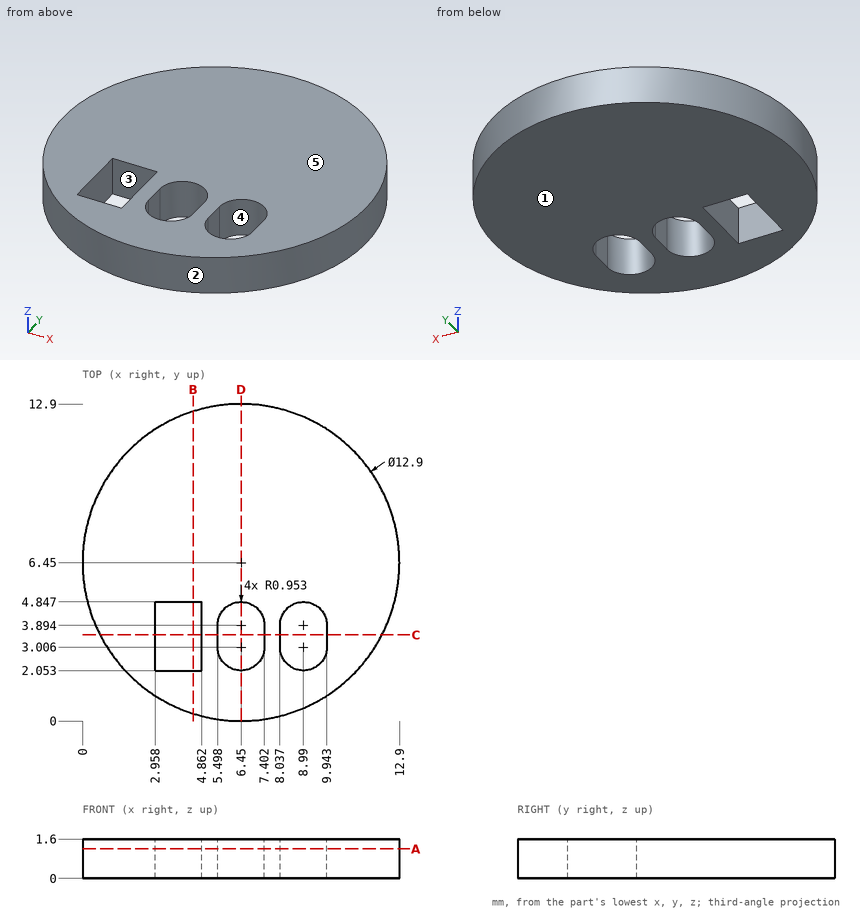
Print and shaded views of the part. All mm, measured from the part's lowest x, y and z. A direction names the side the tool comes from. Coordinates: 2 decimals unless noted, no trailing zeros. Write each loop counter-clockwise with the first axis right and the second up, starting at its lowest first coordinate (ties: lowest second). Pieces come first, ordered by that corner, then holes. Notation, with made-up numbers: (5.25, 76.5) - (27.25, 76.5) arc R5 ccw to (27.25, 82.5) - close; hole circle Ø9 at (83, 19.25). An arc over 180 degrees is marked (long way). One line per question, with ' | ' between items. Start each with the question number.
Q1. Cut at C-C, the plane y = 3.5. List the corners of the cut face in (x, z) (1 decimal).
Q2. Cut at B-B, the plane x = 4.5. List the corners of the cut face in (y, z), then the cut area to 3 significant figures.
Q3. Pin check, flat tips, straight feed: pin 1 (0.5 mm diameter, centred on x = 3.5, z = 1, fed in from -Y); pin 2 (0.7 mm diameter, centred on y = 3.5, z = 0.5, fed in from -X). Stop position of each tip, or through.
Q4. 3-axis set-ups, long thin cutter, end or side, ignore diameter. For the marked faces 4 and 5: which of +Z, -Z, +X, -X, +Y, -Y reach the whole face in a straight line?
Q5. Pull direction Y, two halves, no side cores. Call the marked faces 1, 2 and 3: pulls with the +Y half, pulls with the -Y half, needs draft (parallel to the pull), parting line crosses it, or undercut.
Q6. Drill centre lines: line 1 (X direction, y = 2.25, z = 0.7) (1 decimal); line 2 (X direction, y = 4.5, z = 0.6) (1 decimal); line 3 (Y direction, x = 8.25, z = 1.1) (1 decimal). Where is each one in solid material? Low to high. Write a range as [from, to].
Q7. Cut at D-D, the plane x = 6.45. List the corners of the cut face in (y, z).
Q8. Cut at A-A, the plane z = 1.2. Give the number of separate pieces and of enclosed holes in the cut face, then the cut area to 3 significant figures.
Answer below:
1) outline: (0.7, 0) - (3, 0) - (3, 1.6) - (0.7, 1.6) - close; (4.9, 0) - (5.5, 0) - (5.5, 1.6) - (4.9, 1.6) - close; (7.4, 0) - (8, 0) - (8, 1.6) - (7.4, 1.6) - close; (9.9, 0) - (12.2, 0) - (12.2, 1.6) - (9.9, 1.6) - close
2) outline: (0.3, 0) - (2.05, 0) - (2.05, 1.6) - (0.3, 1.6) - close; (4.85, 0) - (12.6, 0) - (12.6, 1.6) - (4.85, 1.6) - close | area: 15.2 mm^2
3) pin 1: y = 0.59 | pin 2: x = 0.55
4) face 4: +Z, -Z | face 5: +Z, +X, -X, +Y, -Y
5) face 1: needs draft | face 2: parting line crosses it | face 3: undercut
6) line 1: [1.6, 3], [4.9, 5.9], [7, 8.4], [9.6, 11.3] | line 2: [0.3, 3], [4.9, 5.7], [7.2, 8.3], [9.7, 12.6] | line 3: [0.3, 2.4], [4.5, 12.6]
7) outline: (0, 0) - (2.05, 0) - (2.05, 1.6) - (0, 1.6) - close; (4.85, 0) - (12.9, 0) - (12.9, 1.6) - (4.85, 1.6) - close
8) separate pieces: 1 | enclosed holes: 3 | area: 116 mm^2
